from build123d import *

# Parameters (mm, degrees)
SKETCH2_R                    = 1.9668129
SKETCH2_R_2                  = 4
SKETCH2_R_3                  = 1.5
BASE_FLANGE1_DEPTH           = 2
FILLET1_R                    = 4
EDGE_FLANGE1_STRIP_W         = 9.4732
EDGE_FLANGE1_STRIP_H         = 2
EDGE_FLANGE1_STRIP_CUT_DEPTH = 8
EDGE_FLANGE1_DEPTH           = 8
EDGE_FLANGE2_STRIP_W         = 9.4732
EDGE_FLANGE2_STRIP_H         = 2
EDGE_FLANGE2_STRIP_CUT_DEPTH = 8
EDGE_FLANGE2_DEPTH           = 8
EDGE_FLANGE3_STRIP_W         = 9.4732
EDGE_FLANGE3_STRIP_H         = 2
EDGE_FLANGE3_STRIP_CUT_DEPTH = 42
EDGE_FLANGE3_DEPTH           = 42
FILLET2_R                    = 4
FILLET3_R                    = 4
SKETCH16_R                   = 2.15
SKETCH16_R_2                 = 1.5
CUT_EXTRUDE1_DEPTH           = 54.593376456


# Sheet-metal steps are written as plain solids
with BuildPart() as part:
    # Sketch2 → Base-Flange1 (new body)
    with BuildSketch(Plane(origin=(0, 0, 0), x_dir=(1, 0, 0), z_dir=(0, 1, 0))):
        Polygon((-21, 12.815864023), (-29, 12.815864023), (-29, -9.184135977), (-21, -9.184135977), (-21, -15.684135977), (21, -15.684135977), (21, -9.184135977), (29, -9.184135977), (29, 12.815864023), (21, 12.815864023), (21, 9.815864023), (19, 9.815864023), (19, 19.815864023), (-19, 19.815864023), (-19, 9.815864023), (-21, 9.815864023), align=None)
        with Locations(Location((-25, -3.184135977, 0), (0, 0, 270))):
            Circle(SKETCH2_R, mode=Mode.SUBTRACT)
        with Locations(Location((-25, 6.815864023, 0), (0, 0, 270))):
            Circle(SKETCH2_R, mode=Mode.SUBTRACT)
        with Locations(Location((25.409668555, 6.815864023, 0), (0, 0, 270))):
            Circle(SKETCH2_R, mode=Mode.SUBTRACT)
        with Locations(Location((25.409668555, -3.184135977, 0), (0, 0, 270))):
            Circle(SKETCH2_R, mode=Mode.SUBTRACT)
        with Locations(Location((-10.5, 6.815864023, 0), (0, 0, 270))):
            Circle(SKETCH2_R_2, mode=Mode.SUBTRACT)
        with Locations(Location((10.5, 6.815864023, 0), (0, 0, 270))):
            Circle(SKETCH2_R_2, mode=Mode.SUBTRACT)
        with Locations(Location((0, -3.684135977, 0), (0, 0, 270))):
            Circle(SKETCH2_R_2, mode=Mode.SUBTRACT)
        with Locations(Location((-10.5, 13.815864023, 0), (0, 0, 270))):
            Circle(SKETCH2_R_3, mode=Mode.SUBTRACT)
        with Locations(Location((10.5, 13.815864023, 0), (0, 0, 270))):
            Circle(SKETCH2_R_3, mode=Mode.SUBTRACT)
        with Locations(Location((0, -10.684135977, 0), (0, 0, 270))):
            Circle(SKETCH2_R_3, mode=Mode.SUBTRACT)
        with Locations(Location((-3.5, 6.815864023, 0), (0, 0, 270))):
            Circle(SKETCH2_R_3, mode=Mode.SUBTRACT)
        with Locations(Location((-10.5, -0.184135977, 0), (0, 0, 270))):
            Circle(SKETCH2_R_3, mode=Mode.SUBTRACT)
        with Locations(Location((-17.5, 6.815864023, 0), (0, 0, 270))):
            Circle(SKETCH2_R_3, mode=Mode.SUBTRACT)
        with Locations(Location((17.5, 6.815864023, 0), (0, 0, 270))):
            Circle(SKETCH2_R_3, mode=Mode.SUBTRACT)
        with Locations(Location((10.5, -0.184135977, 0), (0, 0, 270))):
            Circle(SKETCH2_R_3, mode=Mode.SUBTRACT)
        with Locations(Location((3.5, 6.815864023, 0), (0, 0, 270))):
            Circle(SKETCH2_R_3, mode=Mode.SUBTRACT)
        with Locations(Location((-7, -3.684135977, 0), (0, 0, 270))):
            Circle(SKETCH2_R_3, mode=Mode.SUBTRACT)
        with Locations(Location((0, 3.315864023, 0), (0, 0, 270))):
            Circle(SKETCH2_R_3, mode=Mode.SUBTRACT)
        with Locations(Location((7, -3.684135977, 0), (0, 0, 270))):
            Circle(SKETCH2_R_3, mode=Mode.SUBTRACT)
    extrude(amount=-BASE_FLANGE1_DEPTH)

    # Fillet1
    fillet1_edges = [part.edges().sort_by_distance(p)[0] for p in [
        (-19, -1, -19.815864023),
        (19, -1, -19.815864023),
        (29, -1, 9.184135977),
        (-29, -1, 9.184135977),
    ]]
    fillet(fillet1_edges, radius=FILLET1_R)

    # Edge-Flange1 strip (across the edge) → Edge-Flange1 strip cut (cut)
    with BuildSketch(Plane(origin=(-21, 0, -12.815864023), x_dir=(0, 0, 1), z_dir=(-1, 0, 0))):
        with Locations((-4, -1)):
            Rectangle(EDGE_FLANGE1_STRIP_W, EDGE_FLANGE1_STRIP_H)
    extrude(amount=EDGE_FLANGE1_STRIP_CUT_DEPTH, mode=Mode.SUBTRACT)

    # Edge-Flange1 section (across the edge) → Edge-Flange1 (add)
    with BuildSketch(Plane(origin=(-21, 0, -12.815864023), x_dir=(0, 0, 1), z_dir=(-1, 0, 0))):
        with BuildLine():
            Line((-2, 0.7366), (-2, 25))
            Line((-2, 25), (0, 25))
            Line((0, 25), (0, 0.7366))
            ThreePointArc((0, 0.7366), (0.215745145, 0.215745145), (0.7366, 0))
            Line((0.7366, 0), (0.7366, -2))
            ThreePointArc((0.7366, -2), (-1.198468417, -1.198468417), (-2, 0.7366))
        make_face()
    extrude(amount=EDGE_FLANGE1_DEPTH)

    # Edge-Flange2 strip (across the edge) → Edge-Flange2 strip cut (cut)
    with BuildSketch(Plane(origin=(29, 0, -12.815864023), x_dir=(0, 0, 1), z_dir=(-1, 0, 0))):
        with Locations((-4, -1)):
            Rectangle(EDGE_FLANGE2_STRIP_W, EDGE_FLANGE2_STRIP_H)
    extrude(amount=EDGE_FLANGE2_STRIP_CUT_DEPTH, mode=Mode.SUBTRACT)

    # Edge-Flange2 section (across the edge) → Edge-Flange2 (add)
    with BuildSketch(Plane(origin=(29, 0, -12.815864023), x_dir=(0, 0, 1), z_dir=(-1, 0, 0))):
        with BuildLine():
            Line((-2, 0.7366), (-2, 25))
            Line((-2, 25), (0, 25))
            Line((0, 25), (0, 0.7366))
            ThreePointArc((0, 0.7366), (0.215745145, 0.215745145), (0.7366, 0))
            Line((0.7366, 0), (0.7366, -2))
            ThreePointArc((0.7366, -2), (-1.198468417, -1.198468417), (-2, 0.7366))
        make_face()
    extrude(amount=EDGE_FLANGE2_DEPTH)

    # Edge-Flange3 strip (across the edge) → Edge-Flange3 strip cut (cut)
    with BuildSketch(Plane(origin=(-21, 0, 15.684135977), x_dir=(0, 0, -1), z_dir=(1, 0, 0))):
        with Locations((-4, -1)):
            Rectangle(EDGE_FLANGE3_STRIP_W, EDGE_FLANGE3_STRIP_H)
    extrude(amount=EDGE_FLANGE3_STRIP_CUT_DEPTH, mode=Mode.SUBTRACT)

    # Edge-Flange3 section (across the edge) → Edge-Flange3 (add)
    with BuildSketch(Plane(origin=(-21, 0, 15.684135977), x_dir=(0, 0, -1), z_dir=(1, 0, 0))):
        with BuildLine():
            Line((-2, 0.7366), (-2, 25))
            Line((-2, 25), (0, 25))
            Line((0, 25), (0, 0.7366))
            ThreePointArc((0, 0.7366), (0.215745145, 0.215745145), (0.7366, 0))
            Line((0.7366, 0), (0.7366, -2))
            ThreePointArc((0.7366, -2), (-1.198468417, -1.198468417), (-2, 0.7366))
        make_face()
    extrude(amount=EDGE_FLANGE3_DEPTH)

    # Fillet2
    fillet2_edges = [part.edges().sort_by_distance(p)[0] for p in [
        (-29, 25, -13.815864023),
        (29, 25, -13.815864023),
    ]]
    fillet(fillet2_edges, radius=FILLET2_R)

    # Fillet3
    fillet3_edges = [part.edges().sort_by_distance(p)[0] for p in [
        (-21, 25, 16.684135977),
        (21, 25, 16.684135977),
    ]]
    fillet(fillet3_edges, radius=FILLET3_R)

    # Sketch16 → Cut-Extrude1 (cut, through all)
    with BuildSketch(Plane.XY.offset(17.684135977)):
        with Locations(Location((-24.2, 17.870640786, 0), (0, 0, 270))):
            Circle(SKETCH16_R)
        with Locations(Location((24.2, 17.870640786, 0), (0, 0, 270))):
            Circle(SKETCH16_R)
        with Locations(Location((-24.2, 6.570640786, 0), (0, 0, 270))):
            Circle(SKETCH16_R)
        with Locations(Location((24.2, 6.570640786, 0), (0, 0, 270))):
            Circle(SKETCH16_R)
        with Locations((-10.25, 12.330953146)):
            Circle(SKETCH16_R_2)
        with Locations((-10.25, 5.330953146)):
            Circle(SKETCH16_R_2)
        with Locations((10.25, 12.330953146)):
            Circle(SKETCH16_R_2)
        with Locations((10.25, 5.330953146)):
            Circle(SKETCH16_R_2)
        with Locations((-17.25, 12.330953146)):
            Circle(SKETCH16_R_2)
        with Locations((-10.25, 19.330953146)):
            Circle(SKETCH16_R_2)
        with Locations((-3.25, 12.330953146)):
            Circle(SKETCH16_R_2)
        with Locations((3.25, 12.330953146)):
            Circle(SKETCH16_R_2)
        with Locations((10.25, 19.330953146)):
            Circle(SKETCH16_R_2)
        with Locations((17.25, 12.330953146)):
            Circle(SKETCH16_R_2)
    extrude(amount=-CUT_EXTRUDE1_DEPTH, mode=Mode.SUBTRACT)


solid = part.part
The listing builds one solid part. Answer for the finished solid, in the listing's coordinates (mm). A direction names the side the tool comes from. Round coordinates to 2 decimals unless told otherwise and drop trailing zeros. Write each loop counter-clockwise with the first axis right and the second up, starting at its lowest first coordinate (ties: lowest second). Pieces come first, ordered by that corner, then holes. Notation, with made-up numbers: (88.5, -4.5) - (138.5, -4.5) arc R22 cw to (138.5, 13.5) - close; hole circle Ø10 at (-14.75, 74). An arc over 180 degrees is marked (long way). Use one line per item in the form item = value. Start each with the question number.
Item 1: A tool of negligible diameter and unlimited length cuts with its end or side. For faces 1 (the flat face through (23, -1, 9.184)), 2 (the flat face through (19, -1, -13)), 3 (the flat face through (0, 13, 15.684)), 4 (the cylindrical face through (-22.39, 5.41, -13.8)), from which of +Z, -Z, +X, -X, +Y, -Y can it reach the whole face along a straight path? Write none if from no direction.
Item 2: A cutting plane is placed at B-B (z = -13.5). Give the number of separate pieces and of enclosed holes in the cut face, plus the area to 3 significant figures.
Item 3: Find the intervals of material crossed by line 1 (Y direction, x = -10, z = 16); line 2 (X direction, y = 10.75, z = -14.5); line 3 (Y direction, x = 25, z = -0.5), in increasing order. Write a range as [from, to].
Item 4: A cutting plane is placed at C-C (x = 0). Write down the section's boundary in (y, z), plus the area to 3 significant figures.
Item 5: Determine the mould class of faces 5 (the cylindrical face through (-8.464, -0.986, 3.359)), 6 (the cylindrical face through (27.859, 23.797, -13.802)), 7 (the flat face through (-23, -1, 9.184)) for opening direction X: +X half, -X half, draft (parallel to the pull), parting line (faces both ways), or undercut.
Item 6: A cutting plane is placed at A-A (y = 9.5). Write down the section's boundary in (x, z).
Item 7: Flat-ended cylindrical pins translate along their axes: pin 1 Ø4 at (x, z) = (10.5, 0.18) entering from +Y; pin 2 Ø12 at (x, y) = (-8.5, 4.5) entering from -Z; pin 3 Ø4 at (x, y) = (15, 5.5) entering from -Z; pin 4 Ø2.5 at (x, y) = (-10.25, 12.33) entering from +Z. Find the tip coordinate at first contact, or state that the pin passes through.
The answers:
q1.face_1 = +Z, +X, +Y, -Y
q1.face_2 = -Z, +Y, -Y
q1.face_3 = -Z, +X, -X, +Y
q1.face_4 = +Z, -Z
q2.separate_pieces = 5
q2.enclosed_holes = 4
q2.area = 425 mm^2
q3.line_1 = [-1.79, 3.85], [6.81, 10.85], [13.81, 17.85], [20.81, 25]
q3.line_2 = [-29, -21], [21, 29]
q3.line_3 = [-2, 0]
q4.outline = (-2, -19.82) - (0, -19.82) - (0, -4.82) - (-2, -4.82) - close; (-2, -1.82) - (0, -1.82) - (0, -0.32) - (-2, -0.32) - close; (-2, 7.68) - (0, 7.68) - (0, 9.18) - (-2, 9.18) - close; (-2, 12.18) - (0, 12.18) - (0, 14.95) arc R0.74 cw to (0.74, 15.68) - (25, 15.68) - (25, 17.68) - (0.74, 17.68) arc R2.74 ccw to (-2, 14.95) - close
q4.area = 95.5 mm^2
q5.face_5 = undercut
q5.face_6 = +X half
q5.face_7 = draft
q6.outline = (-29, -14.82) - (-21, -14.82) - (-21, -12.82) - (-29, -12.82) - close; (-21, 15.68) - (21, 15.68) - (21, 17.68) - (-21, 17.68) - close; (21, -14.82) - (29, -14.82) - (29, -12.82) - (21, -12.82) - close
q7.pin_1 = 0
q7.pin_2 = -19.82
q7.pin_3 = 15.68
q7.pin_4 = through
